Verification items for the finished model (mm, model axes). Face numbers are marked on the shaded views. Give positions to 0.01 mm unless a question says otherwise; leave off trailing zeros. Order: outer loops, then holes, each group sorted by start corner. A loop starts at its lowest first (then second) coordinate and runs counter-clockwise, first axis right, second up.
(1) Mould release check, pull along X, two halves, no side actions. Record for the marked faces 1, 2, 3 and 4: pulls with the +X half, pulls with the -X half, needs draft (parallel to the pull), parting line crosses it, or undercut.
(2) Sectioned sample at C-C on z = 9.9. Record the cut outline in (x, y).
(3) Sectioned sample at D-D on y = 1. Record the cut outline in (x, z).
(4) Gauge pin test, flat end, axial feed: pin 1 (4 mm diameter, centred on x = -6, z = 5.5, fed in from +Y). Record the tip position at first contact, or that the pin passes through.
(5) Sectioned sample at B-B on x = -9. Record the cut outline in (y, z).
(6) Sectioned sample at A-A on y = 8. Record the cut outline in (x, z).
(7) Scan lines: L1, parallel to Z at x = 23.9, y = -1; L2, parallel to X at y = -1.45, z = 20.1; L3, parallel to X at y = 0.5, z = 22. Record each from-to range of solid material in increasing order.
Solid Edge part; units mm, degrees
sketch "Sketch1" plane through (0, 0, 0) normal (0, 0, 1) x (1, 0, 0)
  line L0 (29, -2) -> (29, 18)
  line L1 (27, 18) -> (29, 18)
  line L2 (27, 0) -> (27, 18)
  line L3 (0, 0) -> (27, 0)
  line L4 (0, -2) -> (0, 0)
  line L5 (0, -2) -> (29, -2)
extrude "Protrusion1" add sketch "Sketch1" along normal blind 30
hole "Hole1" at (23.9, -2, 20.1) direction (0, 1, 0) diameter 4.2 end up to next
hole "Hole2" at (23.9, -2, 9.9) direction (0, 1, 0) diameter 4.2 end up to next
sketch "Sketch2" plane through (14.5, -2, 12.5) normal (0, -1, 0) x (1, 0, 0)
  line L0 (-14.5, 12.75) -> (6, 12.75)
  line L1 (6, 12.75) -> (6, -7.75)
  line L2 (6, -7.75) -> (-14.5, -7.75)
  line L3 (-14.5, -7.75) -> (-14.5, 12.75)
  dimension "D1" = 14.5
  dimension "D2" = 6
extrude "Cutout1" cut sketch "Sketch2" against normal up to next
sketch "Sketch3" plane through (29, 8, 15) normal (1, 0, 0) x (0, 1, 0)
  circle A0 centre (0, 0) radius 3.5
extrude "Cutout2" cut sketch "Sketch3" against normal up to next
mirror "Mirror1" about plane through (0, -1, 23.875) normal (-1, 0, 0) of "Protrusion1", "Cutout1", "Hole1", "Hole2"
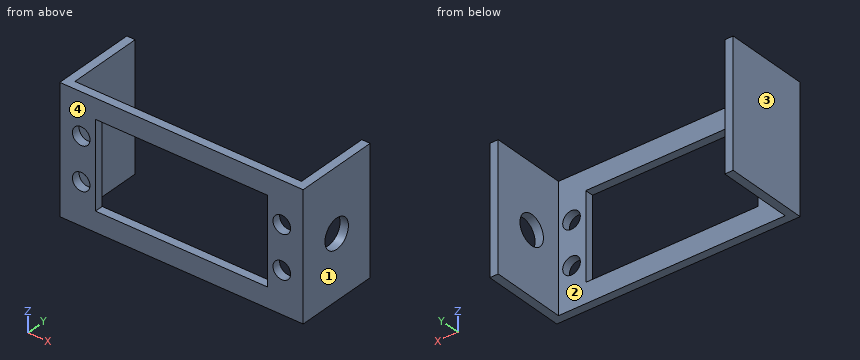
Ans:
1. face 1: pulls with the +X half
1. face 2: undercut
1. face 3: pulls with the -X half
1. face 4: needs draft
2. outline: (-29, -2) - (-26, -2) - (-26, 0) - (-27, 0) - (-27, 18) - (-29, 18) - close; (-21.8, -2) - (-20.5, -2) - (-20.5, 0) - (-21.8, 0) - close; (20.5, -2) - (21.8, -2) - (21.8, 0) - (20.5, 0) - close; (26, -2) - (29, -2) - (29, 18) - (27, 18) - (27, 0) - (26, 0) - close
3. outline: (-29, 0) - (-27, 0) - (-27, 30) - (-29, 30) - close; (27, 0) - (29, 0) - (29, 30) - (27, 30) - close
4. pin 1: stops at y = 0
5. outline: (-2, 0) - (0, 0) - (0, 4.75) - (-2, 4.75) - close; (-2, 25.25) - (0, 25.25) - (0, 30) - (-2, 30) - close
6. outline: (-29, 0) - (-27, 0) - (-27, 30) - (-29, 30) - close; (27, 0) - (29, 0) - (29, 11.5) - (27, 11.5) - close; (27, 18.5) - (29, 18.5) - (29, 30) - (27, 30) - close
7. L1: z = 0 to 7.8, 12 to 18, 22.2 to 30
7. L2: x = -29 to -26, -21.8 to -20.5, 20.5 to 21.8, 26 to 29
7. L3: x = -29 to -27, 27 to 29
